from build123d import *

# Parameters (mm, degrees)
SKETCH1_R           = 1.6
SKETCH1_R_2         = 1.75
SKETCH1_R_3         = 3.95
SKETCH1_R_4         = 12
SKETCH1_R_5         = 3
BOSS_EXTRUDE1_DEPTH = 3


with BuildPart() as part:
    # Sketch1 → Boss-Extrude1 (new body)
    with BuildSketch(Plane(origin=(0, 0, 0), x_dir=(1, 0, 0), z_dir=(0, 1, 0))):
        with BuildLine():
            Line((294.373353, 1022.190294437), (327.907309833, 1022.190294437))
            ThreePointArc((327.907309833, 1022.190294437), (328.157309833, 1022.257281735), (328.340322535, 1022.440294437))
            ThreePointArc((328.340322535, 1022.440294437), (329.126888323, 1022.543848684), (329.023336329, 1021.757282599))
            ThreePointArc((329.023336329, 1021.757282599), (328.840324865, 1021.574270305), (328.773337833, 1021.324271437))
            Line((328.773337833, 1021.324271437), (328.773337833, 1019.690242437))
            ThreePointArc((328.773337833, 1019.690242437), (328.919784442, 1019.336689047), (329.273337833, 1019.190242437))
            Line((329.273337833, 1019.190242437), (334.273335833, 1019.190242437))
            ThreePointArc((334.273335833, 1019.190242437), (334.626889492, 1019.336688397), (334.773336751, 1019.690241519))
            Line((334.773336751, 1019.690241519), (334.773336751, 1021.324268519))
            ThreePointArc((334.773336751, 1021.324268519), (334.706349307, 1021.57426848), (334.523336498, 1021.757281075))
            ThreePointArc((334.523336498, 1021.757281075), (334.419781792, 1022.543846802), (335.206347937, 1022.440295269))
            ThreePointArc((335.206347937, 1022.440295269), (335.389360338, 1022.257283911), (335.639359245, 1022.190297025))
            Line((335.639359245, 1022.190297025), (340.773337745, 1022.190297025))
            Line((340.773337745, 1022.190297025), (340.773337745, 1024.990297025))
            Line((340.773337745, 1024.990297025), (339.423337745, 1024.990297025))
            Line((339.423337745, 1024.990297025), (339.423337745, 1029.190297025))
            Line((339.423337745, 1029.190297025), (340.773337745, 1029.190297025))
            Line((340.773337745, 1029.190297025), (340.773337745, 1032.190297025))
            Line((340.773337745, 1032.190297025), (343.973337745, 1032.190297025))
            Line((343.973337745, 1032.190297025), (343.973337745, 1029.190297025))
            Line((343.973337745, 1029.190297025), (345.323337745, 1029.190297025))
            Line((345.323337745, 1029.190297025), (345.323337745, 1024.990292188))
            Line((345.323337745, 1024.990292188), (343.973337745, 1024.990292188))
            Line((343.973337745, 1024.990292188), (343.973337745, 1022.190292188))
            Line((343.973337745, 1022.190292188), (349.107314245, 1022.190292188))
            ThreePointArc((349.107314245, 1022.190292188), (349.357314245, 1022.257279486), (349.540326947, 1022.440292188))
            ThreePointArc((349.540326947, 1022.440292188), (350.326891976, 1022.543845827), (350.223341741, 1021.75728035))
            ThreePointArc((350.223341741, 1021.75728035), (350.040330277, 1021.574268055), (349.973343245, 1021.324269188))
            Line((349.973343245, 1021.324269188), (349.973343245, 1019.690240188))
            ThreePointArc((349.973343245, 1019.690240188), (350.119789854, 1019.336686797), (350.473343245, 1019.190240188))
            Line((350.473343245, 1019.190240188), (355.473340245, 1019.190240188))
            ThreePointArc((355.473340245, 1019.190240188), (355.826893904, 1019.336686148), (355.973341163, 1019.69023927))
            Line((355.973341163, 1019.69023927), (355.973341163, 1021.32426627))
            ThreePointArc((355.973341163, 1021.32426627), (355.906353816, 1021.574266257), (355.723341079, 1021.757278924))
            ThreePointArc((355.723341079, 1021.757278924), (355.619786681, 1022.543844692), (356.406352785, 1022.44029285))
            ThreePointArc((356.406352785, 1022.44029285), (356.589365364, 1022.257281277), (356.839364571, 1022.190294437))
            Line((356.839364571, 1022.190294437), (372.373340046, 1022.190294437))
            Line((372.373340046, 1022.190294437), (372.373340046, 1072.190301225))
            ThreePointArc((372.373340046, 1072.190301225), (370.908873244, 1075.725833838), (367.373340046, 1077.190299225))
            Line((367.373340046, 1077.190299225), (299.37334805, 1077.190299225))
            ThreePointArc((299.37334805, 1077.190299225), (295.837816019, 1075.725834155), (294.373353, 1072.190301275))
            Line((294.373353, 1072.190301275), (294.373353, 1022.190294437))
        make_face()
        with Locations((366.893344996, 1047.842461747)):
            Circle(SKETCH1_R, mode=Mode.SUBTRACT)
        with Locations((357.873345496, 1071.990299275)):
            Circle(SKETCH1_R_2, mode=Mode.SUBTRACT)
        with Locations((357.873345496, 1040.990299275)):
            Circle(SKETCH1_R_2, mode=Mode.SUBTRACT)
        with Locations((304.373346, 1053.49029927)):
            Circle(SKETCH1_R_3, mode=Mode.SUBTRACT)
        with Locations((342.373345496, 1056.490299275)):
            Circle(SKETCH1_R_4, mode=Mode.SUBTRACT)
        with Locations((326.873345496, 1071.990299275)):
            Circle(SKETCH1_R_2, mode=Mode.SUBTRACT)
        with Locations((326.873345496, 1040.990299275)):
            Circle(SKETCH1_R_2, mode=Mode.SUBTRACT)
        with Locations((317.853347996, 1047.84952041)):
            Circle(SKETCH1_R, mode=Mode.SUBTRACT)
        with Locations((304.373346, 1069.49029927)):
            Circle(SKETCH1_R_5, mode=Mode.SUBTRACT)
        with Locations((304.373346, 1037.49029927)):
            Circle(SKETCH1_R_5, mode=Mode.SUBTRACT)
        with BuildLine():
            Line((365.243389653, 1060.95296097), (365.243389653, 1056.48501097))
            ThreePointArc((365.243389653, 1056.48501097), (365.176400533, 1056.235010504), (364.993385671, 1056.051998658))
            ThreePointArc((364.993385671, 1056.051998658), (364.889836092, 1055.26543287), (365.676401176, 1055.368987799))
            ThreePointArc((365.676401176, 1055.368987799), (365.859413353, 1055.55200075), (366.109412996, 1055.618988627))
            Line((366.109412996, 1055.618988627), (367.677282996, 1055.618988627))
            ThreePointArc((367.677282996, 1055.618988627), (367.927282247, 1055.552001761), (368.110294834, 1055.368990124))
            ThreePointArc((368.110294834, 1055.368990124), (368.896860423, 1055.26543905), (368.793306996, 1056.052004329))
            ThreePointArc((368.793306996, 1056.052004329), (368.610294145, 1056.235017289), (368.543306996, 1056.485017627))
            Line((368.543306996, 1056.485017627), (368.543306996, 1060.952967627))
            ThreePointArc((368.543306996, 1060.952967627), (368.610293862, 1061.202966879), (368.793305499, 1061.385979465))
            ThreePointArc((368.793305499, 1061.385979465), (368.89685718, 1062.172545813), (368.110291294, 1062.068990627))
            ThreePointArc((368.110291294, 1062.068990627), (367.927278767, 1061.885978026), (367.677278996, 1061.818990627))
            Line((367.677278996, 1061.818990627), (366.109410996, 1061.818990627))
            ThreePointArc((366.109410996, 1061.818990627), (365.859411616, 1061.885977015), (365.676398679, 1062.068988302))
            ThreePointArc((365.676398679, 1062.068988302), (364.889832133, 1062.172538478), (364.993388824, 1061.38597279))
            ThreePointArc((364.993388824, 1061.38597279), (365.176401775, 1061.202960613), (365.243389653, 1060.95296097))
        make_face(mode=Mode.SUBTRACT)
        with BuildLine():
            Line((318.637281496, 1061.818997965), (317.069414496, 1061.818997965))
            ThreePointArc((317.069414496, 1061.818997965), (316.819415116, 1061.885984352), (316.636402179, 1062.06899564))
            ThreePointArc((316.636402179, 1062.06899564), (315.849836392, 1062.172545208), (315.953391324, 1061.385980127))
            ThreePointArc((315.953391324, 1061.385980127), (316.136404615, 1061.202967361), (316.203392153, 1060.952966947))
            Line((316.203392153, 1060.952966947), (316.203392153, 1056.485018307))
            ThreePointArc((316.203392153, 1056.485018307), (316.136403033, 1056.235017841), (315.953388171, 1056.052005995))
            ThreePointArc((315.953388171, 1056.052005995), (315.849838592, 1055.265440207), (316.636403676, 1055.368995136))
            ThreePointArc((316.636403676, 1055.368995136), (316.819416286, 1055.552008337), (317.069416496, 1055.618995965))
            Line((317.069416496, 1055.618995965), (318.637286496, 1055.618995965))
            ThreePointArc((318.637286496, 1055.618995965), (318.887285747, 1055.552009098), (319.070298334, 1055.368997461))
            ThreePointArc((319.070298334, 1055.368997461), (319.856863923, 1055.265446387), (319.753310496, 1056.052011666))
            ThreePointArc((319.753310496, 1056.052011666), (319.570297645, 1056.235024626), (319.503310496, 1056.485024964))
            Line((319.503310496, 1056.485024964), (319.503310496, 1060.952974964))
            ThreePointArc((319.503310496, 1060.952974964), (319.570297362, 1061.202974216), (319.753308999, 1061.385986802))
            ThreePointArc((319.753308999, 1061.385986802), (319.85686068, 1062.17255315), (319.070294794, 1062.068997964))
            ThreePointArc((319.070294794, 1062.068997964), (318.887281834, 1061.885985114), (318.637281496, 1061.818997965))
        make_face(mode=Mode.SUBTRACT)
        with BuildLine():
            Line((316.203388653, 1039.193570463), (316.203388653, 1034.725621463))
            ThreePointArc((316.203388653, 1034.725621463), (316.136399531, 1034.475620993), (315.953384663, 1034.292609147))
            ThreePointArc((315.953384663, 1034.292609147), (315.849835095, 1033.506043359), (316.636400176, 1033.609598291))
            ThreePointArc((316.636400176, 1033.609598291), (316.819412786, 1033.792611493), (317.069412996, 1033.85959912))
            Line((317.069412996, 1033.85959912), (318.637282996, 1033.85959912))
            ThreePointArc((318.637282996, 1033.85959912), (318.887282247, 1033.792612254), (319.070294834, 1033.609600616))
            ThreePointArc((319.070294834, 1033.609600616), (319.856860423, 1033.506049543), (319.753306996, 1034.292614822))
            ThreePointArc((319.753306996, 1034.292614822), (319.570294395, 1034.475627349), (319.503306996, 1034.72562712))
            Line((319.503306996, 1034.72562712), (319.503306996, 1039.19357712))
            ThreePointArc((319.503306996, 1039.19357712), (319.570293862, 1039.443576372), (319.753305499, 1039.626588958))
            ThreePointArc((319.753305499, 1039.626588958), (319.856856573, 1040.413154547), (319.070291294, 1040.30960112))
            ThreePointArc((319.070291294, 1040.30960112), (318.887278334, 1040.126588269), (318.637277996, 1040.05960112))
            Line((318.637277996, 1040.05960112), (317.069410996, 1040.05960112))
            ThreePointArc((317.069410996, 1040.05960112), (316.819411616, 1040.126587508), (316.636398679, 1040.309598795))
            ThreePointArc((316.636398679, 1040.309598795), (315.849832892, 1040.413148364), (315.953387824, 1039.626583283))
            ThreePointArc((315.953387824, 1039.626583283), (316.136401025, 1039.443570673), (316.203388653, 1039.193570463))
        make_face(mode=Mode.SUBTRACT)
        with BuildLine():
            Line((368.543303996, 1034.72562712), (368.543303996, 1039.19357712))
            ThreePointArc((368.543303996, 1039.19357712), (368.610290862, 1039.443576372), (368.793302499, 1039.626588958))
            ThreePointArc((368.793302499, 1039.626588958), (368.896853573, 1040.413154547), (368.110288294, 1040.30960112))
            ThreePointArc((368.110288294, 1040.30960112), (367.927275767, 1040.126588519), (367.677275996, 1040.05960112))
            Line((367.677275996, 1040.05960112), (366.109407996, 1040.05960112))
            ThreePointArc((366.109407996, 1040.05960112), (365.859408616, 1040.126587508), (365.676395679, 1040.309598795))
            ThreePointArc((365.676395679, 1040.309598795), (364.889829133, 1040.413148971), (364.993385824, 1039.626583283))
            ThreePointArc((364.993385824, 1039.626583283), (365.176399025, 1039.443570673), (365.243386653, 1039.193570463))
            Line((365.243386653, 1039.193570463), (365.243386653, 1034.725621463))
            ThreePointArc((365.243386653, 1034.725621463), (365.176397531, 1034.475620993), (364.993382663, 1034.292609147))
            ThreePointArc((364.993382663, 1034.292609147), (364.889833095, 1033.506043359), (365.676398176, 1033.609598291))
            ThreePointArc((365.676398176, 1033.609598291), (365.859410353, 1033.792611243), (366.109409996, 1033.85959912))
            Line((366.109409996, 1033.85959912), (367.677279996, 1033.85959912))
            ThreePointArc((367.677279996, 1033.85959912), (367.927279247, 1033.792612254), (368.110291834, 1033.609600616))
            ThreePointArc((368.110291834, 1033.609600616), (368.896857423, 1033.506049543), (368.793303996, 1034.292614822))
            ThreePointArc((368.793303996, 1034.292614822), (368.610291395, 1034.475627349), (368.543303996, 1034.72562712))
        make_face(mode=Mode.SUBTRACT)
    extrude(amount=BOSS_EXTRUDE1_DEPTH)


solid = part.part
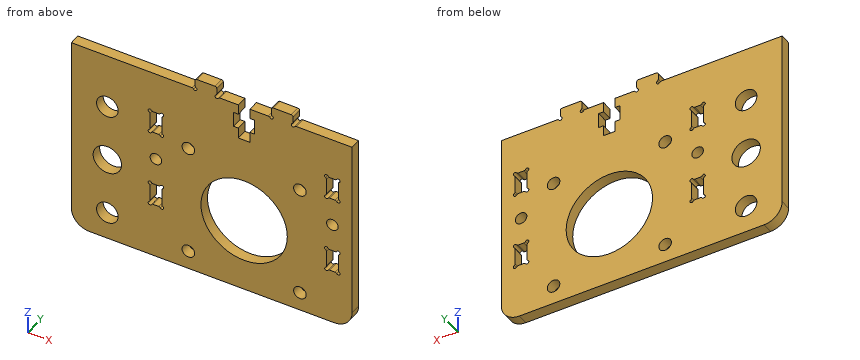
For this review, take the finished solid that the model builds, in its own axes (mm). Round coordinates to 2 decimals unless told otherwise and drop trailing zeros. Loops run counter-clockwise (first coordinate to the right, second up) from the corner with the lowest first, then second, coordinate; pieces in that order, holes last. Notation, with made-up numbers: (-22.75, -7.5) - (13.25, -7.5) arc R15 ccw to (13.25, 3.5) - close; hole circle Ø5 at (33.25, 1.5). An arc over 180 degrees is marked (long way). Answer as CSV lines item,"result".
(1) Consider section C-C on y = 1.4. Give the number of separate pieces and of enclosed holes in the cut face, then the cut area to 3 significant figures.
Checked values:
separate pieces,"1"
enclosed holes,"14"
area,"3,560 mm2"
(2) Consider section B-B on x = 331.5. Give the boundary of the cut face in (y, z), then the cut area to 3 significant figures.
Checked values:
outline,"(0, -1077.19) - (3, -1077.19) - (3, -1061.57) - (0, -1061.57) - close; (0, -1051.41) - (3, -1051.41) - (3, -1019.19) - (0, -1019.19) - close"
area,"144 mm2"
(3) Consider section D-D on x = 310. Give the boundary of the cut face in (y, z).
Checked values:
outline,"(0, -1077.19) - (3, -1077.19) - (3, -1022.19) - (0, -1022.19) - close"
(4) Consider section A-A on z = -1064.5. Give the boundary of the cut face in (x, y), then the cut area to 3 significant figures.
Checked values:
outline,"(294.37, 0) - (333.44, 0) - (333.44, 3) - (294.37, 3) - close; (351.31, 0) - (372.37, 0) - (372.37, 3) - (351.31, 3) - close"
area,"180 mm2"
(5) Wall thickness on line 1 (Z direction, x = 304.5, y = 2.55); line 2 (X direction, y = 0.8, z = -1059); line 3 (X direction, y = 1.6, z = -1051.5): over which ranges is each line inside the solid? List them lowest first.
Checked values:
line 1,"z = -1077.19 to -1072.49, -1066.49 to -1057.44, -1049.54 to -1040.49, -1034.49 to -1022.19"
line 2,"x = 294.37 to 316.2, 319.5 to 330.64, 354.11 to 365.24, 368.54 to 372.37"
line 3,"x = 294.37 to 300.96, 307.79 to 331.46, 353.29 to 372.37"
(6) Insertion check: P1, Ø0.5, axis at y = 1, z = -1021, coming from the -X side; P2, Ø0.6, axis at x = 334.77, z = -1022.19, coming from the -Y side; P3, Ø0.8, axis at x = 367, y = 2, coming from the +Z side; P4, Ø3, axis at x = 347, z = -1041.5, coming from the -Y side. Each pin has a flat end and moves straight along its axis. Give the tip position at first contact, or say it passes through.
Checked values:
P1,"stops at x = 328.77"
P2,"passes through"
P3,"stops at z = -1022.19"
P4,"stops at y = 0"
